Can you work these out from the model? Positions are in its coordinate system, mm. A direction names the side the tool comes from. Round coordinates to 2 decimals unless told otherwise and drop trailing zeros. Write each loop counter-clockwise with the first axis right and the second up, starting at its lowest first coordinate (ties: lowest second). Pieces come first, ordered by that corner, then holes. Notation, with made-up numbers: (42, -14.5) - (56, -14.5) arc R20 ccw to (56, 23.5) - close; hole circle Ø5 at (-19, -25.75). An arc over 180 degrees is marked (long way). One line per item, written item: value. Start each with the question number.
(1) Thinking about a two-plate mould opening in X: for faces 3 (the face through (-91.84, 224.77, -95.8)), 4 (the face through (5.33, 219.526, -95.795)), 5 (the face through (3.9, 5.3, -103.2)), 6 (the face through (100.3, 12.88, 97.61)), which applies, +X half, -X half, draft (parallel to the pull), parting line (faces both ways), or undercut?
(2) I want a section at A-A on y = 198.12. List the corners of the cut face in (x, z) for me.
(3) On a 3-axis mill with a long thin cutter (end or side, diameter ignored), from which of +Z, -Z, +X, -X, +Y, -Y can I reach the whole of each face in a straight line? I mean faces 1 (the face through (104.119, 57, -90)), 2 (the face through (1, 127, -82.917)). Say none if no direction works.
(4) I'm going to push flat-ended pins straight in: pin 1 Ø5 at (x, z) = (48, -8) entering from +Y; pin 2 Ø12 at (x, y) = (-5.5, 97.5) entering from +Z. Where does each tip first touch, or does it pass through?
(5) I want a section at D-D on z = 76. List the corners of the cut face in (x, y) for me.
(6) I want a section at B-B on x = 68. List the corners of the cut face in (y, z) for me.
(7) I want a section at C-C on x = -7. List the corners of the cut face in (y, z) for me.
(8) If I drill on L1, parallel to Y at x = 74, z = 73; L2, parallel to Z at x = 88, y = 153, over which ranges is the centre line in solid material (lowest first)? Write a range as from..to.
from build123d import *

# Parameters (mm, degrees)
SKETCH1_W           = 203.2
SKETCH1_H           = 209.55
BOSS_EXTRUDE2_DEPTH = 25.4
SKETCH2_W           = 203.2
SKETCH2_H           = 25.4
BOSS_EXTRUDE3_DEPTH = 207.01
CUT_EXTRUDE1_REACH  = 211.55
SKETCH3_R           = 21.59
FILLET1_R           = 17.78
FILLET2_R           = 25.4
FILLET3_R           = 12.7


with BuildPart() as part:
    # Sketch1 → Boss-Extrude2 (new body)
    with BuildSketch(Plane(origin=(0, 0, 0), x_dir=(1, 0, 0), z_dir=(0, 1, 0))):
        with Locations((2.519008264, 3.542355372)):
            Rectangle(SKETCH1_W, SKETCH1_H)
    extrude(amount=BOSS_EXTRUDE2_DEPTH)

    # Sketch2 → Boss-Extrude3 (add)
    with BuildSketch(Plane(origin=(0, 25.4, 0), x_dir=(1, 0, 0), z_dir=(0, 1, 0))):
        with Locations((2.519008264, 95.617355372)):
            Rectangle(SKETCH2_W, SKETCH2_H)
    extrude(amount=BOSS_EXTRUDE3_DEPTH)

    # Sketch3 → Cut-Extrude1 (cut, up to next)
    with BuildSketch(Plane(origin=(0, 0, -108.317355372), x_dir=(-1, 0, 0), z_dir=(0, 0, -1)), mode=Mode.PRIVATE) as cut_extrude1_sk1:
        with Locations((-2.519008264, 198.12)):
            Circle(SKETCH3_R)
    cut_extrude1_tool1 = extrude(cut_extrude1_sk1.sketch, amount=-CUT_EXTRUDE1_REACH, mode=Mode.PRIVATE) & part.part
    add(cut_extrude1_tool1.solids().sort_by_distance((2.519008, 198.12, -108.317355))[0], mode=Mode.SUBTRACT)

    # Fillet1
    fillet1_edges = [part.edges().sort_by_distance(p)[0] for p in [
        (2.519008264, 0, -108.317355372),
    ]]
    fillet(fillet1_edges, radius=FILLET1_R)

    # Fillet2
    fillet2_edges = [part.edges().sort_by_distance(p)[0] for p in [
        (-99.080991736, 232.41, -95.617355372),
        (104.119008264, 232.41, -95.617355372),
    ]]
    fillet(fillet2_edges, radius=FILLET2_R)

    # Fillet3
    fillet3_edges = [part.edges().sort_by_distance(p)[0] for p in [
        (104.119008264, 12.7, 101.232644628),
        (-99.080991736, 12.7, 101.232644628),
    ]]
    fillet(fillet3_edges, radius=FILLET3_R)


solid = part.part
Established:
1. face 3: -X half
1. face 4: undercut
1. face 5: draft
1. face 6: +X half
2. outline: (-99.08, -108.32) - (-19.07, -108.32) - (-19.07, -82.92) - (-99.08, -82.92) - close; (24.11, -108.32) - (104.12, -108.32) - (104.12, -82.92) - (24.11, -82.92) - close
3. face 1: +Z, -Z, +X, +Y, -Y
3. face 2: +Z, +X, -X, +Y
4. pin 1: y = 25.4
4. pin 2: z = -82.92
5. outline: (-99.08, 0) - (104.12, 0) - (104.12, 25.4) - (-99.08, 25.4) - close
6. outline: (0, -90.54) arc R17.78 ccw to (17.78, -108.32) - (232.41, -108.32) - (232.41, -82.92) - (25.4, -82.92) - (25.4, 101.23) - (0, 101.23) - close
7. outline: (0, -90.54) arc R17.78 ccw to (17.78, -108.32) - (178.74, -108.32) - (178.74, -82.92) - (25.4, -82.92) - (25.4, 101.23) - (0, 101.23) - close; (217.5, -108.32) - (232.41, -108.32) - (232.41, -82.92) - (217.5, -82.92) - close
8. L1: 0..25.4
8. L2: -108.32..-82.92
